from build123d import *

# Parameters (mm, degrees)
SKETCH1_R           = 2.5
BOSS_EXTRUDE1_DEPTH = 4
FILLET2_R           = 3


with BuildPart() as part:
    # Sketch1 → Boss-Extrude1 (new body)
    with BuildSketch(Plane.XY):
        with BuildLine():
            Line((15.011053362, 49.830662375), (3.838692378, 83.622901822))
            Line((3.838692378, 83.622901822), (4.361186649, 84.509770663))
            ThreePointArc((4.361186649, 84.509770663), (11.04786713, 90.978220722), (10.57313596, 81.686979022))
            Line((10.57313596, 81.686979022), (18.898131325, 55.650415498))
            Line((18.898131325, 55.650415498), (18.969275223, 55.368960637))
            ThreePointArc((18.969275223, 55.368960637), (24.583713079, 48.126504338), (15.45509163, 48.928599175))
            Line((15.45509163, 48.928599175), (15.011053362, 49.830662375))
        make_face()
        with Locations((8.979351439, 86.426161535)):
            Circle(SKETCH1_R, mode=Mode.SUBTRACT)
        with Locations((20.194596002, 50.521426317)):
            Circle(SKETCH1_R, mode=Mode.SUBTRACT)
    extrude(amount=BOSS_EXTRUDE1_DEPTH)

    # Fillet2
    fillet2_edges = [part.edges().sort_by_distance(p)[0] for p in [
        (18.969275223, 55.368960637, 2),
        (10.57313596, 81.686979022, 2),
    ]]
    fillet(fillet2_edges, radius=FILLET2_R)


solid = part.part
Design review of the part built by this model. Coordinates are the model's own, in mm. A direction names the side the tool comes from. Round coordinates to 2 decimals unless told otherwise and drop trailing zeros. Loops run counter-clockwise (first coordinate to the right, second up) from the corner with the lowest first, then second, coordinate; pieces in that order, holes last. Notation, with made-up numbers: (-29.75, 57.25) -> (-6.75, 57.25) arc R26 cw to (-6.75, 85.25) -> close; hole circle Ø4 at (81, 43.25). An arc over 180 degrees is marked (long way). Use one line per item in the form item = value. Start each with the question number.
Q1. We need section D-D on y = 77. Give the boundary of the cut face in (x, z), then the cut area to 3 significant figures.
Q2. For pin 1 Ø1 at (y, z) = (86, 2) entering from +X; pin 2 Ø2 at (x, y) = (17, 53.5) entering from -Z; pin 3 Ø1.5 at (y, z) = (66, 1) entering from +X, all flat-tipped, find the tip position at first contact; note any pin that passes through.
Q3. We need section B-B on y = 87. Give the boundary of the cut face in (x, z).
Q4. We need section A-A on x = 10. Give the boundary of the cut face in (y, z).
Q5. Wall thickness on line 1 along X through (y, z) = (86.5, 2.35); line 2 along X through (y, z) = (88, 3.5); line 3 along Y through (x, z) = (20.5, 1.4): over which ranges is each line inside the solid? List them lowest first. Write a range as [from, to].
Q6. Machinability: for faces 1 (the face through (10, 91.32, 1.97)), 2 (the face through (4.096, 84.06, 1.972)), 3 (the face through (14.746, 68.636, 1.972)), which of the approach directions +Z, -Z, +X, -X, +Y, -Y give a long, thin tool a straight path to every point of the face, cutting with its end or side? Answer none if there is none.
Q7. We need section C-C on z = 2.8. State how many separate pieces and enclosed holes the cut face has, then the cut area to 3 significant figures.
Q8. Draft analysis for pull direction Y (two halves, no side actions). For faces 4 (the face through (24.165, 47.483, 1.972)), 5 (the face through (13, 69, 0)), 6 (the face through (11.28, 81.18, 2.03)), state which applies: +Y half, -Y half, draft (parallel to the pull), parting line (faces both ways), or undercut.
Calculated:
q1.outline = (6.03, 0) -> (12.07, 0) -> (12.07, 4) -> (6.03, 4) -> close
q1.area = 24.2 mm²
q2.pin_1 = 13.98
q2.pin_2 = 0
q2.pin_3 = 15.83
q3.outline = (4.01, 0) -> (6.55, 0) -> (6.55, 4) -> (4.01, 4) -> close; (11.41, 0) -> (13.95, 0) -> (13.95, 4) -> (11.41, 4) -> close
q4.outline = (64.99, 0) -> (84.14, 0) -> (84.14, 4) -> (64.99, 4) -> close; (88.71, 0) -> (91.32, 0) -> (91.32, 4) -> (88.71, 4) -> close
q5.line_1 = [3.98, 6.48], [11.48, 13.98]
q5.line_2 = [4.23, 7.04], [10.92, 13.73]
q5.line_3 = [45.53, 48.04], [53, 55.54]
q6.face_1 = +Z, -Z
q6.face_2 = +Z, -Z, -X
q6.face_3 = +Z, -Z, +X
q7.separate_pieces = 1
q7.enclosed_holes = 2
q7.area = 290 mm²
q8.face_4 = parting line
q8.face_5 = draft
q8.face_6 = undercut
